from build123d import *

# Parameters (mm, degrees)
BOSS_EXTRUDE1_DEPTH = 9.525
BOSS_EXTRUDE2_DEPTH = 4.7625
CUT_EXTRUDE1_DEPTH  = 1.778
FILLET1_R           = 1.524


with BuildPart() as part:
    # Sketch2 → Boss-Extrude1 (new body)
    with BuildSketch(Plane(origin=(0, 0, 0), x_dir=(1, 0, 0), z_dir=(0, 1, 0))):
        with BuildLine():
            Line((8.64, 8.4876), (-8.64, 8.4876))
            Line((-8.64, 8.4876), (-8.64, -8.4876))
            Line((-8.64, -8.4876), (8.64, -8.4876))
            Line((8.64, -8.4876), (8.64, -3.3655))
            Line((8.64, -3.3655), (0.921517153, -3.500226619))
            ThreePointArc((0.921517153, -3.500226619), (-3.6195, 0), (0.921517153, 3.500226619))
            Line((0.921517153, 3.500226619), (8.64, 3.3655))
            Line((8.64, 3.3655), (8.64, 8.4876))
        make_face()
    extrude(amount=BOSS_EXTRUDE1_DEPTH)

    # Sketch3 → Boss-Extrude2 (add)
    with BuildSketch(Plane(origin=(0, 9.525, 0), x_dir=(1, 0, 0), z_dir=(0, 1, 0))):
        with BuildLine():
            Line((11.18, 3.3655), (11.18, 11.0276))
            Line((11.18, 11.0276), (-11.18, 11.0276))
            Line((-11.18, 11.0276), (-11.18, -11.0276))
            Line((-11.18, -11.0276), (11.18, -11.0276))
            Line((11.18, -11.0276), (11.18, -3.3655))
            Line((11.18, -3.3655), (8.64, -3.3655))
            Line((8.64, -3.3655), (0.921517153, -3.500226619))
            ThreePointArc((0.921517153, -3.500226619), (-3.6195, 0), (0.921517153, 3.500226619))
            Line((0.921517153, 3.500226619), (8.64, 3.3655))
            Line((8.64, 3.3655), (11.18, 3.3655))
        make_face()
    extrude(amount=BOSS_EXTRUDE2_DEPTH)

    # Sketch4 → Cut-Extrude1 (cut)
    with BuildSketch(Plane(origin=(0, 6.477, 0), x_dir=(-1, 0, 0), z_dir=(0, -1, 0))):
        with BuildLine():
            Line((3.970210665, 3.447011476), (8.64, 3.447011476))
            Line((8.64, 3.447011476), (8.64, 8.4876))
            Line((8.64, 8.4876), (-8.64, 8.4876))
            Line((-8.64, 8.4876), (-8.64, 3.3655))
            Line((-8.64, 3.3655), (-3.970210665, 3.447011476))
            ThreePointArc((-3.970210665, 3.447011476), (0, 5.2578), (3.970210665, 3.447011476))
        make_face()
        with BuildLine():
            Line((3.970210665, -3.447011476), (8.64, -3.447011476))
            Line((8.64, -3.447011476), (8.64, -8.4876))
            Line((8.64, -8.4876), (-8.64, -8.4876))
            Line((-8.64, -8.4876), (-8.64, -3.3655))
            Line((-8.64, -3.3655), (-3.970210665, -3.447011476))
            ThreePointArc((-3.970210665, -3.447011476), (0, -5.2578), (3.970210665, -3.447011476))
        make_face()
    extrude(amount=CUT_EXTRUDE1_DEPTH, mode=Mode.SUBTRACT)

    # Fillet1
    fillet1_edges = [part.edges().sort_by_distance(p)[0] for p in [
        (8.64, 8.001, 8.4876),
        (-8.64, 8.001, 8.4876),
        (-8.64, 8.001, -8.4876),
        (8.64, 8.001, -8.4876),
        (11.18, 11.90625, -3.3655),
        (11.18, 11.90625, -11.0276),
        (-11.18, 11.90625, -11.0276),
        (-11.18, 11.90625, 11.0276),
        (11.18, 11.90625, 11.0276),
        (11.18, 11.90625, 3.3655),
        (8.64, 2.3495, -3.3655),
        (8.64, 2.3495, 3.3655),
        (8.64, 2.3495, 8.4876),
        (-8.64, 2.3495, 8.4876),
        (-8.64, 2.3495, -8.4876),
        (8.64, 2.3495, -8.4876),
    ]]
    fillet(fillet1_edges, radius=FILLET1_R)


solid = part.part
The listing builds one solid part. Answer for the finished solid, in the listing's coordinates (mm). A direction names the side the tool comes from. Coordinates: 2 decimals unless noted, no trailing zeros. Order: outer loops, then holes, each group sorted by start corner. A loop starts at its lowest first (then second) coordinate and runs counter-clockwise, first axis right, second up. Notation, with made-up numbers: M 7.5,-6.75 L 42.5,-6.75 A28 ccw 42.5,18.25 Z; hole C 33.5,84.25 d1. An arc over 180 degrees is marked long. Use CSV: the item, a comma, the result in double quotes.
Q1. Section D-D (x = 4.5) is taken. Determine the outline of the cut face in (y, z) (1 decimal), then the cut area to 3 significant figures.
Here are the results:
outline,"M 0,-8.5 L 4.7,-8.5 L 4.7,-3.4 L 0,-3.4 Z; M 0,3.4 L 4.7,3.4 L 4.7,8.5 L 0,8.5 Z; M 6.5,-8.5 L 9.5,-8.5 L 9.5,-11 L 14.3,-11 L 14.3,-3.4 L 6.5,-3.4 Z; M 6.5,3.4 L 14.3,3.4 L 14.3,11 L 9.5,11 L 9.5,8.5 L 6.5,8.5 Z"
area,"151 mm2"
Q2. Determine the mould class of faces 6 (the flat face through (-6, 6, -3.447)), 7 (the cylindrical face through (10.72, 11.94, 3.8)), 8 (the cylindrical face through (10.745, 11.94, 10.569)) for opening direction Z: pulls with the +Z half, pulls with the -Z half, needs draft (parallel to the pull), parting line crosses it, or undercut.
Here are the results:
face 6,"pulls with the -Z half"
face 7,"undercut"
face 8,"pulls with the +Z half"
Q3. Section A-A (x = 0) is taken. Determine the outline of the cut face in (y, z) (1 decimal).
Here are the results:
outline,"M 0,-8.5 L 4.7,-8.5 L 4.7,-5.3 L 6.5,-5.3 L 6.5,-8.5 L 9.5,-8.5 L 9.5,-11 L 14.3,-11 L 14.3,-3.6 L 0,-3.6 Z; M 0,3.6 L 14.3,3.6 L 14.3,11 L 9.5,11 L 9.5,8.5 L 6.5,8.5 L 6.5,5.3 L 4.7,5.3 L 4.7,8.5 L 0,8.5 Z"
Q4. Section B-B (x = -5) is taken. Determine the outline of the cut face in (y, z) (1 decimal), then the cut area to 3 significant figures.
Here are the results:
outline,"M 0,-8.5 L 4.7,-8.5 L 4.7,-3.4 L 6.5,-3.4 L 6.5,-8.5 L 9.5,-8.5 L 9.5,-11 L 14.3,-11 L 14.3,11 L 9.5,11 L 9.5,8.5 L 6.5,8.5 L 6.5,3.4 L 4.7,3.4 L 4.7,8.5 L 0,8.5 Z"
area,"249 mm2"
Q5. Given pin 1 Ø0.6 at (y, z) = (3, 6.5) entering from +X; pin 2 Ø4 at (x, y) = (-1, 2.5) entering from +Z; pin 3 Ø0.9 at (x, y) = (2, 8) entering from -Z, each flat-ended and moving along its own axis, determine where each tip first touches the part or whether it passes through.
Here are the results:
pin 1,"x = 8.64"
pin 2,"z = 8.49"
pin 3,"z = -8.49"
Q6. Straight lines are drawn through the part: L1, parallel to Y at x = 5, z = -3.5; L2, parallel to Z at x = 0, y = 7.5; L3, parallel to Z at x = 0, y = 10.75. For each, find the intervals that lie inside material, in ascending order.
Here are the results:
L1,"0 to 4.7, 6.48 to 14.29"
L2,"-8.49 to -3.62, 3.62 to 8.49"
L3,"-11.03 to -3.62, 3.62 to 11.03"
Q7. A tool of negligible diameter and unlimited length cuts with its end or side. For faces 1 (the flat face through (-9, 9.525, 1)), 2 (the flat face through (-8.64, 5, 0)), 3 (the cylindrical face through (8.182, 2.382, 8.053)), 4 (the cylindrical face through (8.205, 2.382, -8.029)), 5 (the cylindrical face through (10.745, 11.94, -3.824)), from which of +Z, -Z, +X, -X, +Y, -Y can it reach the whole face along a straight path? Write none if from no direction.
Here are the results:
face 1,"-Y"
face 2,"+Z, -Z, -X, -Y"
face 3,"+Z, +X, -Y"
face 4,"-Z, +X, -Y"
face 5,"+X, +Y, -Y"
Q8. Section C-C (y = 5) is taken. Determine the outline of the cut face in (x, z), then the cut area to 3 significant figures.
Here are the results:
outline,"M -8.64,-3.45 L -3.97,-3.45 A5.26 ccw 3.97,-3.45 L 0.92,-3.5 A3.62 cw long 0.92,3.5 L 3.97,3.45 A5.26 ccw -3.97,3.45 L -8.64,3.45 Z"
area,"58.5 mm2"
